from build123d import *

# Parameters (mm, degrees)
EXTRUDE_1_DEPTH     = 6
CUT_EXTRUDE_2_DEPTH = 4


with BuildPart() as part:
    # Эскиз1 → Вытянуть1 (new body)
    with BuildSketch(Plane(origin=(0, 0, 0), x_dir=(1, 0, 0), z_dir=(0, 1, 0))):
        Polygon((-12, 0), (-56, 0), (-56, 23.893685267), (-74.88648833, 23.893685267), (-74.88648833, 76.106314733), (-56, 76.106314733), (-56, 100), (-12, 100), align=None)
    extrude(amount=EXTRUDE_1_DEPTH)

    # Эскиз2 → Вытянуть2 (cut)
    with BuildSketch(Plane.XZ):
        Polygon((-56, -5), (-12, -5), (-12, -95), (-56, -95), (-56, -73.28325794), (-74.88648833, -73.28325794), (-74.88648833, -26.71674206), (-56, -26.71674206), align=None)
    extrude(amount=-CUT_EXTRUDE_2_DEPTH, mode=Mode.SUBTRACT)


solid = part.part
Can you work these out from the model? Positions are in its coordinate system, mm. A direction names the side the tool comes from. Give positions to 0.01 mm unless a question says otherwise; leave off trailing zeros. Write each loop counter-clockwise with the first axis right and the second up, starting at its lowest first coordinate (ties: lowest second). Pieces come first, ordered by that corner, then holes. Notation, with made-up numbers: (-13.5, 83.5) -> (24.5, 83.5) arc R23 ccw to (24.5, 92.5) -> close; hole circle Ø7 at (14.25, 64.5). An arc over 180 degrees is marked (long way). Answer as a JSON object with one key per item and string values. Group by question number.
Item 1: Please list where these lines run through material, in increasing order: line 1 (Z direction, x = -55, y = 2.4); line 2 (Z direction, x = -71, y = 2.45); line 3 (Y direction, x = -62, z = -63). Write a range as [from, to].
Item 2: For faces 1 (the face through (-34, 2, -5)), 2 (the face through (-66, 3, -76.106)), 3 (the face through (-56, 2, -25)), which set-ups out of +Z, -Z, +X, -X, +Y, -Y let a thin tool reach every point of the face, with its end or its side?
Item 3: Suppose I cut it at A-A (y = 2.65). Please give me the cut outline in (x, z).
Item 4: I'm going to push flat-ended pins straight in: P1, Ø1.8, axis at x = -63, y = 3.5, coming from the -Z side; P2, Ø2.5, axis at y = 1.5, z = -75.5, coming from the +X side; P3, Ø1.8, axis at y = 2.5, z = -87, coming from the -X side; P4, Ø2, axis at x = -69.5, y = 2, coming from the +Z side. Where does each tip first touch, or does it pass through?
Item 5: Suppose I cut it at D-D (x = -58). Please give me the cut outline in (y, z), plus the area to 3 significant figures.
Item 6: Suppose I cut it at C-C (z = -53.5). Please give me the cut outline in (x, y).
Item 7: Suppose I cut it at B-B (x = -16). Please give me the cut outline in (y, z), plus the area to 3 significant figures.
Findings:
{
 "1": {"line 1": "z = [-100, -95], [-5, 0]", "line 2": "z = [-76.11, -73.28], [-26.72, -23.89]", "line 3": "y = [4, 6]"},
 "2": {"face 1": "+X, -X, -Y", "face 2": "-Z, -X, +Y, -Y", "face 3": "+X, -Y"},
 "3": {"outline": "(-74.89, -76.11) -> (-56, -76.11) -> (-56, -73.28) -> (-74.89, -73.28) -> close; (-74.89, -26.72) -> (-56, -26.72) -> (-56, -23.89) -> (-74.89, -23.89) -> close; (-56, -100) -> (-12, -100) -> (-12, -95) -> (-56, -95) -> close; (-56, -5) -> (-12, -5) -> (-12, 0) -> (-56, 0) -> close"},
 "4": {"P1": "stops at z = -76.11", "P2": "stops at x = -56", "P3": "passes through", "P4": "stops at z = -23.89"},
 "5": {"outline": "(0, -76.11) -> (6, -76.11) -> (6, -23.89) -> (0, -23.89) -> (0, -26.72) -> (4, -26.72) -> (4, -73.28) -> (0, -73.28) -> close", "area": "127 mm²"},
 "6": {"outline": "(-74.89, 4) -> (-12, 4) -> (-12, 6) -> (-74.89, 6) -> close"},
 "7": {"outline": "(0, -100) -> (6, -100) -> (6, 0) -> (0, 0) -> (0, -5) -> (4, -5) -> (4, -95) -> (0, -95) -> close", "area": "240 mm²"}
}
